```python
from build123d import *

# Parameters (mm, degrees)
SKETCH1_W           = 21.082
SKETCH1_H           = 21.082
BOSS_EXTRUDE1_DEPTH = 6.35
BOSS_EXTRUDE2_DEPTH = 11.811
SCALE1_SCALE        = 1.02


with BuildPart() as part:
    # Sketch1 → Boss-Extrude1 (new body)
    with BuildSketch(Plane(origin=(0, 0, 0), x_dir=(1, 0, 0), z_dir=(0, 1, 0))):
        Rectangle(SKETCH1_W, SKETCH1_H)
    extrude(amount=BOSS_EXTRUDE1_DEPTH)

    # Sketch3 → Boss-Extrude2 (add, symmetric)
    with BuildSketch(Plane(origin=(0, 0, 0), x_dir=(0, 0, -1), z_dir=(1, 0, 0))):
        with BuildLine():
            Line((-11.811, 6.35), (11.811, 6.35))
            ThreePointArc((11.811, 6.35), (0, 18.161), (-11.811, 6.35))
        make_face()
    extrude(amount=BOSS_EXTRUDE2_DEPTH, both=True)


with BuildPart() as part_1:
    # Scale1: scaled about (0, 8.473688703, 0)
    add(part.part.scale(SCALE1_SCALE).moved(Location((0, -0.169473774, 0))))


solid = part_1.part
```
Geometry check sheet. Reference: the model listing, model coordinates, mm. A direction names the side the tool comes from. Round coordinates to 2 decimals unless told otherwise and drop trailing zeros. Order: outer loops, then holes, each group sorted by start corner. A loop starts at its lowest first (then second) coordinate and runs counter-clockwise, first axis right, second up. Notation, with made-up numbers: (-24.5, 72.5) - (29.5, 72.5) arc R22 cw to (29.5, 79.5) - close; hole circle Ø11 at (72.5, -14.5). An arc over 180 degrees is marked (long way). Use a Markdown table: item, result. Add a question column.
1) Thickness scan on line 1 along X through (y, z) = (5.5, -10.5); line 2 along Y through (x, z) = (-1, -5.5); line 3 along Y through (x, z) = (-3, 4). Record the ranges inside material, lowest first.
2) Set-up check for faces 1 (the flat face through (12.047, 11, 0)), 2 (the flat face through (-10.752, 3, 0)), 3 (the flat face through (0, 3, -10.752)), 4 (the flat face through (0, 3, 10.752)), 5 (the flat face through (10.752, 3, 0)): record each of +Z, -Z, +X, -X, +Y, -Y from which the full face is reachable in a straight line by a thin tool's end or side.
3) Section check C-C (z = -9). Record the cut outline in (x, y), then the cut area to 3 significant figures.
4) Gauge pin test, flat ends, axial feed: P1, Ø8, axis at x = 7.5, y = 16.5, coming from the -Z side; P2, Ø10, axis at x = 9, z = -9.5, coming from the +Y side; P3, Ø3, axis at x = -3.5, z = -7, coming from the +Y side. Record the tip position at first contact, or that the pin passes through.
5) Section check B-B (x = -4.5). Record the cut outline in (y, z).
6) Section check A-A (z = 0). Record the cut outline in (x, y), then the cut area to 3 significant figures.
7) Section check D-D (y = 12). Record the cut outline in (x, z), then the cut area to 3 significant figures.
Established:
| question | item | result |
|---|---|---|
| 1 | line 1 | -10.75 to 10.75 |
| 1 | line 2 | -0.17 to 17.03 |
| 1 | line 3 | -0.17 to 17.67 |
| 2 | face 1 | +Z, -Z, +X, +Y, -Y |
| 2 | face 2 | +Z, -Z, -X, -Y |
| 2 | face 3 | -Z, +X, -X, -Y |
| 2 | face 4 | +Z, +X, -X, -Y |
| 2 | face 5 | +Z, -Z, +X, -Y |
| 3 | outline | (-12.05, 6.31) - (-10.75, 6.31) - (-10.75, -0.17) - (10.75, -0.17) - (10.75, 6.31) - (12.05, 6.31) - (12.05, 14.32) - (-12.05, 14.32) - close |
| 3 | area | 332 mm2 |
| 4 | P1 | z = -10.33 |
| 4 | P2 | y = 17.48 |
| 4 | P3 | y = 17.03 |
| 5 | outline | (-0.17, -10.75) - (6.31, -10.75) - (6.31, -12.05) arc R12.05 ccw to (6.31, 12.05) - (6.31, 10.75) - (-0.17, 10.75) - close |
| 6 | outline | (-12.05, 6.31) - (-10.75, 6.31) - (-10.75, -0.17) - (10.75, -0.17) - (10.75, 6.31) - (12.05, 6.31) - (12.05, 18.35) - (-12.05, 18.35) - close |
| 6 | area | 430 mm2 |
| 7 | outline | (-12.05, -10.62) - (12.05, -10.62) - (12.05, 10.62) - (-12.05, 10.62) - close |
| 7 | area | 512 mm2 |
